```python
from build123d import *

# Parameters (mm, degrees)
F0_W     = 138.4936049581
F0_H     = 77.3329418153
F0_R     = 19.9688682615
F1_DEPTH = 50.8
F2_R     = 5.08
F3_R     = 5.08
F4_T     = -2.54


# Not quite as in the source:
# - a shell that OpenCascade refuses in one call is made with other operations: the cavity is built on its own and cut out


with BuildPart() as f1:
    # F0 (on Front) → F1 (new body)
    with BuildSketch(Plane.XZ):
        with Locations((-2.6111938059, 14.1139933839)):
            Rectangle(F0_W, F0_H)
        with Locations((9.2974901199, 16.3193047047)):
            Circle(F0_R, mode=Mode.SUBTRACT)
    extrude(amount=F1_DEPTH)

    # F2
    f2_edges = [f1.edges().sort_by_distance(p)[0] for p in [
        (66.635609, 0, 14.113993),
        (-2.611194, 0, 52.780464),
        (-71.857996, 0, 14.113993),
        (-2.611194, 0, -24.552478),
        (-10.671378, 0, 16.319305),
        (-10.671378, -50.8, 16.319305),
    ]]
    fillet(f2_edges, radius=F2_R)

    # F3
    f3_edges = [f1.edges().sort_by_distance(p)[0] for p in [
        (-2.611194, -50.8, -24.552478),
        (-71.857996, -50.8, 14.113993),
        (-2.611194, -50.8, 52.780464),
        (66.635609, -50.8, 14.113993),
    ]]
    fillet(f3_edges, radius=F3_R)

    # F4: a shell. OpenCascade refuses it in one call, so the cavity is built on its own and cut out:
    # the body offset inwards by the wall thickness, plus a prism from it out through each open face.
    f4_core = offset(f1.part, amount=F4_T, mode=Mode.PRIVATE)
    f4_exits = [f4_core.faces().sort_by_distance(p)[0] for p in [
        (-2.611194, -48.26, -18.023971),
    ]]
    add(f4_core, mode=Mode.SUBTRACT)
    extrude(f4_exits, amount=-F4_T, mode=Mode.SUBTRACT)


solid = f1.part
```
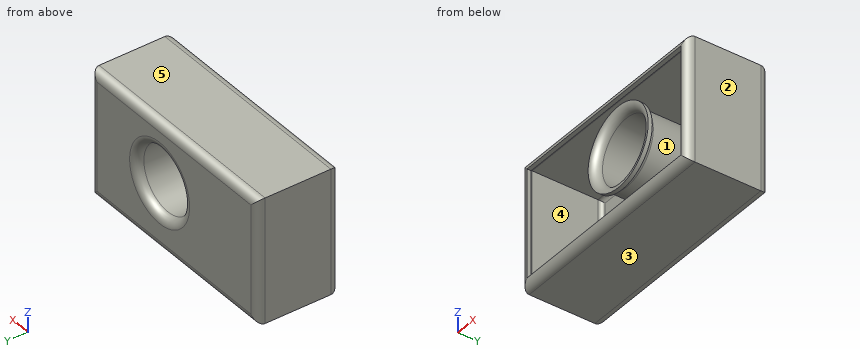
For this review, take the finished solid that the model builds, in its own axes (mm). Face numbers are marked on the shaded views. A direction names the side the tool comes from. Round coordinates to 2 decimals unless told otherwise and drop trailing zeros. Order: outer loops, then holes, each group sorted by start corner. A loop starts at its lowest first (then second) coordinate and runs counter-clockwise, first axis right, second up. Notation, with made-up numbers: (-36.5, -22.75) -> (-6.5, -22.75) arc R23 ccw to (-6.5, -1.75) -> close; hole circle Ø8 at (76, 57). An arc over 180 degrees is marked (long way). Use a Markdown table: item, result.
Item 1: Take a section at B-B (z = 45). State the section outline as (x, y) points.
Resolved:
| item | result |
|---|---|
| outline | (-71.86, -45.72) arc R5.08 ccw to (-66.78, -50.8) -> (-66.78, -48.26) arc R2.54 cw to (-69.32, -45.72) -> (-69.32, -5.08) arc R2.54 cw to (-66.78, -2.54) -> (61.56, -2.54) arc R2.54 cw to (64.1, -5.08) -> (64.1, -45.72) arc R2.54 cw to (61.56, -48.26) -> (61.56, -50.8) arc R5.08 ccw to (66.64, -45.72) -> (66.64, -5.08) arc R5.08 ccw to (61.56, 0) -> (-66.78, 0) arc R5.08 ccw to (-71.86, -5.08) -> close |
Item 2: Take a section at C-C (x = -28). State the section outline as (y, z) points.
Resolved:
| item | result |
|---|---|
| outline | (-50.8, -19.47) arc R5.08 ccw to (-45.72, -24.55) -> (-5.08, -24.55) arc R5.08 ccw to (0, -19.47) -> (0, 47.7) arc R5.08 ccw to (-5.08, 52.78) -> (-45.72, 52.78) arc R5.08 ccw to (-50.8, 47.7) -> (-48.26, 47.7) arc R2.54 cw to (-45.72, 50.24) -> (-5.08, 50.24) arc R2.54 cw to (-2.54, 47.7) -> (-2.54, -19.47) arc R2.54 cw to (-5.08, -22.01) -> (-45.72, -22.01) arc R2.54 cw to (-48.26, -19.47) -> close |
Item 3: For line 1 along X through (y, z) = (-35.5, 45.5); line 2 along Z through (x, y) = (49, -24); line 3 along X through (y, z) = (-15.5, 2), list the stretches that pass through material, from the lowest coordinate up. Write a range as [from, to].
Resolved:
| item | result |
|---|---|
| line 1 | x = [-71.86, -69.32], [64.1, 66.64] |
| line 2 | z = [-24.55, -22.01], [50.24, 52.78] |
| line 3 | x = [-71.86, -69.32], [-8.07, -4.62], [23.22, 26.66], [64.1, 66.64] |
Item 4: Machinability: for the marked faces 4 and 5, which of the approach directions +Z, -Z, +X, -X, +Y, -Y give a long, thin tool a straight path to every point of the face, cutting with its end or side? Answer none if there is none.
Resolved:
| item | result |
|---|---|
| face 4 | none |
| face 5 | +Z, +X, -X, +Y, -Y |
Item 5: Take a section at A-A (y = -26). State the section outline as (x, z) points.
Resolved:
| item | result |
|---|---|
| outline | (-71.86, -24.55) -> (66.64, -24.55) -> (66.64, 52.78) -> (-71.86, 52.78) -> close; circle Ø45.02 at (9.3, 16.32); hole (-69.32, -22.01) -> (64.1, -22.01) -> (64.1, 50.24) -> (-69.32, 50.24) -> close; hole circle Ø39.94 at (9.3, 16.32) |
Item 6: Draft analysis for pull direction Z (two halves, no side actions). For the marked faces 1, 2 and 3, state which applies: +Z half, -Z half, draft (parallel to the pull), parting line (faces both ways), or undercut.
Resolved:
| item | result |
|---|---|
| face 1 | undercut |
| face 2 | draft |
| face 3 | -Z half |
Item 7: For pin 1 (2 mm diameter, centred on y = -50, z = 31, fed in from +X); pin 2 (0.8 mm diameter, centred on x = 9, y = -49.5, fed in from +Z); pin 3 (2 mm diameter, centred on x = -4, y = -49.5, fed in from -Z), all flat-tipped, find the tip position at first contact; note any pin that passes through.
Resolved:
| item | result |
|---|---|
| pin 1 | stops at x = 65.43 |
| pin 2 | stops at z = 51.49 |
| pin 3 | stops at z = -23.72 |
